Build history of the part. All positions in model axes, mm. Face numbers are marked on the shaded views. A direction names the side the tool comes from. Round coordinates to 2 decimals unless told otherwise and drop trailing zeros. Order: outer loops, then holes, each group sorted by start corner. A loop starts at its lowest first (then second) coordinate and runs counter-clockwise, first axis right, second up. Notation, with made-up numbers: M 5,-15 L 41,-15 A12 ccw 41,1 Z; hole C 10,-32 d11. An arc over 180 degrees is marked long. One line per question, with ' | ' between items. Start each with the question number.
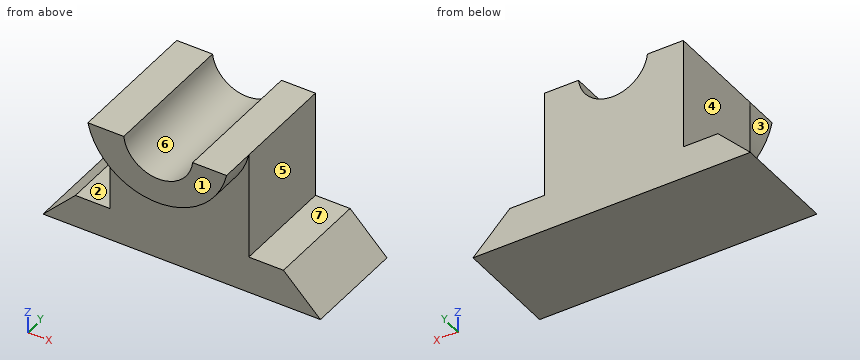
from build123d import *

# Parameters (mm, degrees)
F1_DEPTH = 30
F3_DEPTH = 10
F5_DEPTH = 40.001


with BuildPart() as f1:
    # F0 (on Front) → F1 (new body)
    with BuildSketch(Plane.XZ):
        Polygon((9.355192, 9.355192), (0, 0), (80, 0), (69.355192, 10.644808), (59.355192, 10.644808), (59.355192, 41.47071), (19.355192, 41.47071), (19.355192, 9.355192), align=None)
    extrude(amount=F1_DEPTH)

    # F2 (on face) → F3 (join)
    with BuildSketch(Plane.XZ.offset(30)):
        with BuildLine():
            Line((59.355192, 41.47071), (19.355192, 41.47071))
            ThreePointArc((19.355192, 41.47071), (39.355192, 25.341718), (59.355192, 41.47071))
        make_face()
    extrude(amount=F3_DEPTH)

    # F4 (on face) → F5 (cut, through all)
    with BuildSketch(Plane.XZ.offset(40)):
        with BuildLine():
            Line((49.568015, 41.47071), (29.695006, 41.47071))
            ThreePointArc((29.695006, 41.47071), (39.631511, 32.595821), (49.568015, 41.47071))
        make_face()
    extrude(amount=-F5_DEPTH, mode=Mode.SUBTRACT)


solid = f1.part
Item 1: Cut at A-A on y = -6.5. Write the cut outline in (x, z) (3 decimals), then the cut area to 3 significant figures.
Item 2: Cut at B-B on z = 29.5. Write the cut outline in (x, y), then the cut area to 3 significant figures.
Item 3: Cut at C-C on z = 38. Write the cut outline in (x, y), then the cut area to 3 significant figures.
Item 4: Two-plate mould, pull along X, no slides. Class the marked faces 4, 5, 6 and 7: +X half, -X half, draft (parallel to the pull), parting line (faces both ways), or undercut.
Item 5: Tool access for the marked faces 1, 2 and 3: list every direction of +Z, -Z, +X, -X, +Y, -Y with a clear straight run to the whole face (end or side of a thin tool).
Item 6: Wall check: line 1 along Z through (x, y) = (13.5, -5.5); line 2 along Y through (x, z) = (57.5, 18.5); line 3 along Z through (x, y) = (65.5, -5.5). Give the ranges that are in metal, low to high. Write a range as [from, to].
Item 7: Cut at D-D on x = 40. Write the cut outline in (y, z).
Item 8: Flat gauge pins, fed straight in: pin 1 (8 mm diameter, centred on x = 20.5, z = 6, fed in from -Y); pin 2 (1 mm diameter, centred on x = 43, y = -25.5, fed in from +Z); pin 3 (9 mm diameter, centred on y = -9, z = 21.5, fed in from -X). Where does each tip first touch, or does it go through?
Results found:
1) outline: M 0,0 L 80,0 L 69.355,10.645 L 59.355,10.645 L 59.355,41.471 L 49.568,41.471 A10 cw 29.695,41.471 L 19.355,41.471 L 19.355,9.355 L 9.355,9.355 Z | area: 1,820 mm^2
2) outline: M 19.36,-30 L 26.99,-30 L 26.99,-40 L 51.72,-40 L 51.72,-30 L 59.36,-30 L 59.36,0 L 19.36,0 Z | area: 1,450 mm^2
3) outline: M 19.36,-30 L 20.44,-30 L 20.44,-40 L 30.75,-40 L 30.75,0 L 19.36,0 Z; M 48.51,-40 L 58.27,-40 L 58.27,-30 L 59.36,-30 L 59.36,0 L 48.51,0 Z | area: 868 mm^2
4) face 4: -X half | face 5: +X half | face 6: undercut | face 7: draft
5) face 1: +Z, -Z, +X, -X, -Y | face 2: +Z, -X, +Y, -Y | face 3: -Z, -Y
6) line 1: z = [0, 9.36] | line 2: y = [-30, 0] | line 3: z = [0, 10.64]
7) outline: M -40,25.35 L -30,25.35 L -30,0 L 0,0 L 0,32.6 L -40,32.6 Z
8) pin 1: stops at y = -30 | pin 2: stops at z = 33.37 | pin 3: stops at x = 19.36
